```python
from build123d import *

# Parameters (mm, degrees)
SKETCH1_R           = 11
BOSS_EXTRUDE1_DEPTH = 14.8
SKETCH2_R           = 5.16
BOSS_EXTRUDE2_DEPTH = 8
SKETCH3_R           = 3.175
BOSS_EXTRUDE3_DEPTH = 12.8
SKETCH4_R           = 0.75
BOSS_EXTRUDE4_DEPTH = 2.1


with BuildPart() as part:
    # Sketch1 → Boss-Extrude1 (new body)
    with BuildSketch(Plane(origin=(0, 0, 0), x_dir=(1, 0, 0), z_dir=(0, 1, 0))):
        Circle(SKETCH1_R)
    extrude(amount=BOSS_EXTRUDE1_DEPTH)

    # Sketch2 → Boss-Extrude2 (add)
    with BuildSketch(Plane.XZ):
        Circle(SKETCH2_R)
    extrude(amount=BOSS_EXTRUDE2_DEPTH)

    # Sketch3 → Boss-Extrude3 (add)
    with BuildSketch(Plane(origin=(0, -8, 0), x_dir=(-1, 0, 0), z_dir=(0, -1, 0))):
        Circle(SKETCH3_R)
    extrude(amount=BOSS_EXTRUDE3_DEPTH)

    # Sketch4 → Boss-Extrude4 (add)
    with BuildSketch(Plane.XZ):
        with Locations((7.9, 0)):
            Circle(SKETCH4_R)
    extrude(amount=BOSS_EXTRUDE4_DEPTH)


solid = part.part
```
Work out the finished part from the listing and answer in its coordinate system (mm). A direction names the side the tool comes from. Round coordinates to 2 decimals unless told otherwise and drop trailing zeros. Order: outer loops, then holes, each group sorted by start corner. A loop starts at its lowest first (then second) coordinate and runs counter-clockwise, first axis right, second up.
Q1. The mould has two halves that part along X. Classify faces 4 (the cylindrical face through (0.69, -14.31, 3.1)), 5 (the cylindrical face through (8.615, -1.035, 0.225)), 6 (the flat face through (0, 14.8, 0)): pulls with the +X half, pulls with the -X half, needs draft (parallel to the pull), parting line crosses it, or undercut.
Solution:
face 4: parting line crosses it
face 5: undercut
face 6: needs draft
Q2. A cutting plane is placed at D-D, the plane x = 7.9. Determine the outline of the cut face in (y, z).
Solution:
outline: (-2.1, -0.75) - (0, -0.75) - (0, -7.65) - (14.8, -7.65) - (14.8, 7.65) - (0, 7.65) - (0, 0.75) - (-2.1, 0.75) - close
Q3. A cutting plane is placed at B-B, the plane z = 0. Determine the outline of the cut face in (x, y) (3 decimals), then the cut area to 3 significant figures.
Solution:
outline: (-11, 0) - (-5.16, 0) - (-5.16, -8) - (-3.175, -8) - (-3.175, -20.8) - (3.175, -20.8) - (3.175, -8) - (5.16, -8) - (5.16, 0) - (7.15, 0) - (7.15, -2.1) - (8.65, -2.1) - (8.65, 0) - (11, 0) - (11, 14.8) - (-11, 14.8) - close
area: 493 mm2
Q4. A cutting plane is placed at A-A, the plane x = 0. Determine the outline of the cut face in (y, z) (3 decimals), then the cut area to 3 significant figures.
Solution:
outline: (-20.8, -3.175) - (-8, -3.175) - (-8, -5.16) - (0, -5.16) - (0, -11) - (14.8, -11) - (14.8, 11) - (0, 11) - (0, 5.16) - (-8, 5.16) - (-8, 3.175) - (-20.8, 3.175) - close
area: 489 mm2
Q5. Given pin 1 Ø1.6 at (x, z) = (8, 0.5) entering from -Y; pin 2 Ø2 at (y, z) = (-4.5, -0.5) entering from -X; pin 3 Ø1.5 at (y, z) = (-6.5, -7.5) entering from -X; pin 4 Ø3 at (x, y) = (7.5, 4.5) entering from -Z, each flat-ended and moving along its own axis, determine where each tip first touches the part or whether it passes through.
Solution:
pin 1: stops at y = -2.1
pin 2: stops at x = -5.16
pin 3: passes through
pin 4: stops at z = -9.22
Q6. Find the intervals of material crossed by line 1 along Y through (x, z) = (-2, -9); line 2 along Y through (x, z) = (-3.25, -3); line 3 along X through (y, z) = (1.5, -8), in increasing order.
Solution:
line 1: y = 0 to 14.8
line 2: y = -8 to 14.8
line 3: x = -7.55 to 7.55
Q7. A tool of negligible diameter and unlimited length cuts with its end or side. For faces 1 (the flat face through (8, -2.1, 0)), 2 (the flat face through (2, 0, 5)), 3 (the flat face through (0, -20.8, 0)), from which of +Z, -Z, +X, -X, +Y, -Y can it reach the whole face along a straight path? Write none if from no direction.
Solution:
face 1: +Z, -Z, +X, -Y
face 2: -Y
face 3: +Z, -Z, +X, -X, -Y
Q8. A cutting plane is placed at C-C, the plane y = 5.5. Determine the outline of the cut face in (x, z).
Solution:
outline: circle Ø22 at (0, 0)
